Geometry check sheet. Reference: the model listing, model coordinates, mm. Face numbers are marked on the shaded views. A direction names the side the tool comes from. Coordinates: 2 decimals unless noted, no trailing zeros. Loops run counter-clockwise (first coordinate to the right, second up) from the corner with the lowest first, then second, coordinate; pieces in that order, holes last.
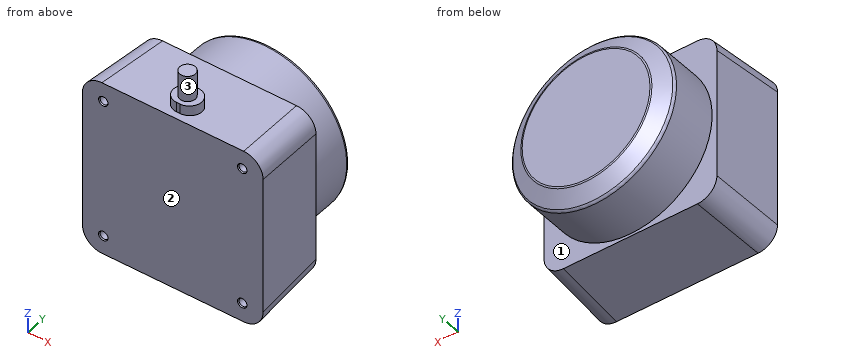
from build123d import *

# Parameters (mm, degrees)
SKETCH1_W           = 55.65
SKETCH1_H           = 54.22051571
BOSS_EXTRUDE1_DEPTH = 23
BOSS_EXTRUDE1_TAPER = 3
SKETCH2_R           = 25.15
BOSS_EXTRUDE2_DEPTH = 18
CHAMFER1_SIZE       = 3
CHAMFER1_SIZE2      = 5.196152423
BOSS_EXTRUDE3_DEPTH = 30
SKETCH4_R           = 2.375
BOSS_EXTRUDE4_DEPTH = 8
SKETCH5_R           = 1.25
CUT_EXTRUDE1_DEPTH  = 5
CHAMFER2_SIZE       = 0.2
CHAMFER2_SIZE2      = 0.346410162
FILLET1_R           = 6
FILLET2_R           = 1


with BuildPart() as part:
    # Sketch1 → Boss-Extrude1 (new body)
    with BuildSketch(Plane(origin=(0, 0, 0), x_dir=(1, 0, 0), z_dir=(0, 1, 0))):
        Rectangle(SKETCH1_W, SKETCH1_H)
    extrude(amount=BOSS_EXTRUDE1_DEPTH, taper=BOSS_EXTRUDE1_TAPER)

    # Sketch2 → Boss-Extrude2 (add)
    with BuildSketch(Plane(origin=(0, 23, 0), x_dir=(1, 0, 0), z_dir=(0, 1, 0))):
        with Locations(Location((0, 0, 0), (0, 0, 270))):
            Circle(SKETCH2_R)
    extrude(amount=BOSS_EXTRUDE2_DEPTH)

    # Chamfer1
    chamfer1_edges = [part.edges().sort_by_distance(p)[0] for p in [
        (0, 41, -25.15),
    ]]
    chamfer1_side = [part.faces().sort_by_distance(p)[0] for p in [
        (0, 32, -25.15),
    ]]
    chamfer(chamfer1_edges, length=CHAMFER1_SIZE, length2=CHAMFER1_SIZE2, reference=chamfer1_side[0])

    # Sketch3 → Boss-Extrude3 (add)
    with BuildSketch(Plane.XY):
        with BuildLine():
            Line((0.55, 2.25), (-0.55, 2.25))
            ThreePointArc((-0.55, 2.25), (-4.3, 6), (-0.55, 9.75))
            Line((-0.55, 9.75), (0.55, 9.75))
            ThreePointArc((0.55, 9.75), (4.3, 6), (0.55, 2.25))
        make_face()
    extrude(amount=BOSS_EXTRUDE3_DEPTH)

    # Sketch4 → Boss-Extrude4 (add)
    with BuildSketch(Plane.XY.offset(30)):
        with Locations((0, 6)):
            Circle(SKETCH4_R)
    extrude(amount=BOSS_EXTRUDE4_DEPTH)

    # Sketch5 → Cut-Extrude1 (cut)
    with BuildSketch(Plane.XZ):
        with Locations(Location((-21.4, 21.4, 0), (0, 0, 270))):
            Circle(SKETCH5_R)
        with Locations(Location((21.4, 21.4, 0), (0, 0, 270))):
            Circle(SKETCH5_R)
        with Locations(Location((21.4, -21.4, 0), (0, 0, 270))):
            Circle(SKETCH5_R)
        with Locations(Location((-21.4, -21.4, 0), (0, 0, 270))):
            Circle(SKETCH5_R)
    extrude(amount=-CUT_EXTRUDE1_DEPTH, mode=Mode.SUBTRACT)

    # Chamfer2
    chamfer2_edges = [part.edges().sort_by_distance(p)[0] for p in [
        (-21.4, 0, -20.15),
        (21.4, 0, -20.15),
        (21.4, 0, 22.65),
        (-21.4, 0, 22.65),
    ]]
    chamfer2_side = [part.faces().sort_by_distance(p)[0] for p in [
        (0, 0, 0),
    ]]
    chamfer(chamfer2_edges, length=CHAMFER2_SIZE, length2=CHAMFER2_SIZE2, reference=chamfer2_side[0])

    # Fillet1
    fillet1_edges = [part.edges().sort_by_distance(p)[0] for p in [
        (-27.222310538, 11.5, -26.507568393),
        (27.222310538, 11.5, -26.507568393),
        (27.222310538, 11.5, 26.507568393),
        (-27.222310538, 11.5, 26.507568393),
    ]]
    fillet(fillet1_edges, radius=FILLET1_R)

    # Fillet2
    fillet2_edges = [part.edges().sort_by_distance(p)[0] for p in [
        (0, 41, -19.953847577),
        (0, 38, -25.15),
    ]]
    fillet(fillet2_edges, radius=FILLET2_R)


solid = part.part
1) Access from +Z, -Z, +X, -X, +Y, -Y to the whole of each face (thin tool, end or side, straight path). Record for the marked faces 1, 2 and 3.
Data:
face 1: +Y
face 2: +Z, -Z, +X, -X, -Y
face 3: +Z
2) Section check A-A on z = 31.5. Record the cut outline in (x, y) (3 decimals), and give its area (3 significant figures).
Data:
outline: circle Ø4.75 at (0, 6)
area: 17.7 mm2
3) Depth check by flat-ended pin: pin 1 (1.2 mm diameter, centred on x = 21.5, z = -21.5, fed in from -Y); pin 2 (5 mm diameter, centred on x = -2.5, z = 9, fed in from -Y); pin 3 (3 mm diameter, centred on x = 3.5, y = 13.5, fed in from +Z); pin 4 (1.2 mm diameter, centred on x = 0, z = 29, fed in from +Y). Enter the tip coordinate at first touch or a pass-through.
Data:
pin 1: stops at y = 5
pin 2: stops at y = 0
pin 3: stops at z = 26.48
pin 4: stops at y = 9.75
4) Material ranges on probe 1 along X at (y, z) = (2, 21); probe 2 along Z at (x, y) = (-21, 2); probe 3 along Z at (x, y) = (0, 25.5), recorded low to high.
Data:
probe 1: x = -27.72 to -22.58, -20.22 to 20.22, 22.58 to 27.72
probe 2: z = -27.01 to -22.58, -20.22 to 20.22, 22.58 to 27.01
probe 3: z = -25.15 to 25.15
